Check sheet for the modelled part. Datum: model origin and axes. Units: mm. Give positions to 0.01 mm unless a question says otherwise; leave off trailing zeros. Order: outer loops, then holes, each group sorted by start corner. A loop starts at its lowest first (then second) coordinate and runs counter-clockwise, first axis right, second up.
Item 1: Sectioned sample at A-A on y = 10. Record the boundary of the cut face in (x, z), and give its area (3 significant figures).
Item 2: Sectioned sample at C-C on x = 56. Record the boundary of the cut face in (y, z).
Item 3: Material ranges on line 1 along X through (y, z) = (-8.5, -15); line 2 along X through (y, z) = (7.5, -10); line 3 along Z through (x, y) = (24, -13.5), recorded low to high.
Item 4: Sectioned sample at B-B on x = 43.5. Record the boundary of the cut face in (y, z), and give its area (3 significant figures).
Item 5: Gauge pin test, flat ends, axial feed: P1, Ø5, axis at x = 37.5, z = -13.5, coming from the -Y side; P2, Ø2, axis at x = 43, y = -10, coming from the +Z side; P3, Ø4, axis at x = 51.5, y = -9.5, coming from the +Z side. Record the tip position at first contact, or that the pin passes through.
Autodesk Inventor part; units mm, degrees
ref_plane "工作平面1" through (10, 18, 0) normal (-0.3451, -0.6637, -0.6637) x (0.8872, 0, -0.4614)
ref_plane "YZ Plane" through (0, 0, 0) normal (1, 0, 0) x (0, 1, 0)
ref_plane "XZ Plane" through (0, 0, 0) normal (0, 1, 0) x (-1, 0, 0)
sketch "草圖1" plane through (0, 0, 0) normal (0, 1, 0) x (-1, 0, 0)
  line L0 (0, 0) -> (-60, 0)
  line L1 (-60, 0) -> (-60, -36)
  line L2 (-60, -36) -> (0, -36)
  line L3 (0, -36) -> (0, 0)
  dimension "d0" = 60
  dimension "d1" = 36
extrude "擠出1" add sketch "草圖1" along normal mid plane 36
sketch "草圖2" plane through (0, 18, 0) normal (0, 1, 0) x (1, 0, 0)
  line L0 (0, 0) -> (60, 0)
  line L1 (10, 0) -> (60, 6)
  line L2 (60, 0) -> (60, 36)
  dimension "d4" = 10
  dimension "d5" = 30
extrude "擠出2" cut sketch "草圖2" against normal blind 40
sketch "草圖3" plane through (60, -18, -36) normal (1, 0, 0) x (0, 0, -1)
  line L0 (-30, 16) -> (-10, 36)
  line L1 (0, 36) -> (-36, 36)
  line L2 (-30, 36) -> (-30, 0)
  point P0 (-36, 18)
  dimension "d8" = 20
  dimension "d9" = 20
ref_plane "工作平面1" through (10, 18, 0) normal (-0.3451, -0.6637, -0.6637) x (0.8872, 0, -0.4614)
sketch "草圖4" plane through (10, 18, 0) normal (-0.3451, -0.6637, -0.6637) x (0.8872, 0, -0.4614)
  line L0 (-15.1543, -12.3218) -> (93.717, -12.3218)
  line L1 (93.717, -12.3218) -> (93.717, 28.8166)
  line L2 (93.717, 28.8166) -> (-15.1543, 28.8166)
  line L3 (-15.1543, 28.8166) -> (-15.1543, -12.3218)
  point P0 (-8.8722, 10.4027)
extrude "擠出3" cut sketch "草圖4" against normal blind 40
mirror "鏡射1" about plane through (0, 0, 0) normal (0, 1, 0) of "擠出3"
properties part number "3"
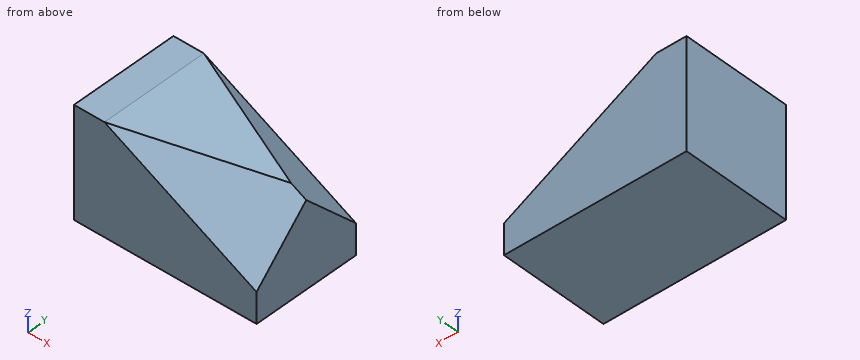
Report:
1. outline: (0, -36) - (60, -36) - (60, -18) - (29.99, -2.4) - (10, 0) - (0, 0) - close
1. area: 1,830 mm2
2. outline: (-18, -36) - (18, -36) - (18, -23.92) - (0, -5.92) - (-18, -23.92) - close
3. line 1: x = 0 to 57.11
3. line 2: x = 0 to 49.42
3. line 3: z = -36 to -2.78
4. outline: (-18, -36) - (18, -36) - (18, -17.42) - (4.6, -4.02) - (-4.6, -4.02) - (-18, -17.42) - close
4. area: 972 mm2
5. P1: stops at y = -18
5. P2: stops at z = -8.03
5. P3: stops at z = -10.83
